```python
from build123d import *

# Parameters (mm, degrees)
BOSS_EXTRUDE1_DEPTH = 5
SKETCH2_R           = 2.5
CUT_EXTRUDE1_DEPTH  = 5
SKETCH3_R           = 3
CUT_EXTRUDE2_DEPTH  = 3
SKETCH4_R           = 2.5
BOSS_EXTRUDE2_DEPTH = 3


with BuildPart() as part:
    # Sketch1 → Boss-Extrude1 (new body)
    with BuildSketch(Plane.XY):
        Polygon((-87.5, 70), (-87.5, 65), (-92.5, 65), (-92.5, -65), (-87.5, -65), (-87.5, -70), (87.5, -70), (87.5, -65), (92.5, -65), (92.5, 65), (87.5, 65), (87.5, 70), align=None)
    extrude(amount=BOSS_EXTRUDE1_DEPTH)

    # Sketch2 → Cut-Extrude1 (cut)
    with BuildSketch(Plane.XY.offset(5)):
        with Locations((-52.5, -25)):
            Circle(SKETCH2_R)
        with Locations((-52.5, 25)):
            Circle(SKETCH2_R)
    extrude(amount=-CUT_EXTRUDE1_DEPTH, mode=Mode.SUBTRACT)

    # Sketch3 → Cut-Extrude2 (cut)
    with BuildSketch(Plane(origin=(0, 0, 0), x_dir=(-1, 0, 0), z_dir=(0, 0, -1))):
        with Locations((52.5, 25)):
            Circle(SKETCH3_R)
        with Locations((52.5, -25)):
            Circle(SKETCH3_R)
    extrude(amount=-CUT_EXTRUDE2_DEPTH, mode=Mode.SUBTRACT)

    # Sketch4 → Boss-Extrude2 (add)
    with BuildSketch(Plane.XY.offset(5)):
        with Locations(Location((58, 0, 0), (0, 0, 180))):
            Circle(SKETCH4_R)
        with BuildLine():
            Line((51.105600012, -5.785088487), (50.339555569, -6.427876097))
            ThreePointArc((50.339555569, -6.427876097), (58, -10), (65.660444431, -6.427876097))
            Line((65.660444431, -6.427876097), (64.894399988, -5.785088487))
            ThreePointArc((64.894399988, -5.785088487), (58, -9), (51.105600012, -5.785088487))
        make_face()
        with BuildLine():
            Line((68.724622204, -8.999026536), (69.490666647, -9.641814145))
            ThreePointArc((69.490666647, -9.641814145), (58, -15), (46.509333353, -9.641814145))
            Line((46.509333353, -9.641814145), (47.275377796, -8.999026536))
            ThreePointArc((47.275377796, -8.999026536), (58, -14), (68.724622204, -8.999026536))
        make_face()
        with BuildLine():
            Line((43.445155581, 12.212964584), (42.679111138, 12.855752194))
            ThreePointArc((42.679111138, 12.855752194), (58, 20), (73.320888862, 12.855752194))
            Line((73.320888862, 12.855752194), (72.554844419, 12.212964584))
            ThreePointArc((72.554844419, 12.212964584), (58, 19), (43.445155581, 12.212964584))
        make_face()
        with BuildLine():
            Line((47.275377796, 8.999026536), (46.509333353, 9.641814145))
            ThreePointArc((46.509333353, 9.641814145), (58, 15), (69.490666647, 9.641814145))
            Line((69.490666647, 9.641814145), (68.724622204, 8.999026536))
            ThreePointArc((68.724622204, 8.999026536), (58, 14), (47.275377796, 8.999026536))
        make_face()
        with BuildLine():
            Line((51.105600012, 5.785088487), (50.339555569, 6.427876097))
            ThreePointArc((50.339555569, 6.427876097), (58, 10), (65.660444431, 6.427876097))
            Line((65.660444431, 6.427876097), (64.894399988, 5.785088487))
            ThreePointArc((64.894399988, 5.785088487), (58, 9), (51.105600012, 5.785088487))
        make_face()
        with BuildLine():
            Line((43.445155581, -12.212964584), (42.679111138, -12.855752194))
            ThreePointArc((42.679111138, -12.855752194), (58, -20), (73.320888862, -12.855752194))
            Line((73.320888862, -12.855752194), (72.554844419, -12.212964584))
            ThreePointArc((72.554844419, -12.212964584), (58, -19), (43.445155581, -12.212964584))
        make_face()
    extrude(amount=BOSS_EXTRUDE2_DEPTH)


solid = part.part
```
Input: part model. Units: mm. Frame: model coordinates. A direction names the side the tool comes from. Give positions to 0.01 mm unless a question says otherwise; leave off trailing zeros. Order: outer loops, then holes, each group sorted by start corner. A loop starts at its lowest first (then second) coordinate and runs counter-clockwise, first axis right, second up. Notation, with made-up numbers: M 71,15 L 112,15 A31 ccw 112,41 Z; hole C 83.5,43.5 d7. An arc over 180 degrees is marked long. Return JSON: item names as keys, results as strings.
Item 1: Pull-direction query (Y, two-part tool) for faces 1 (the flat face through (-90, -65, 2)), 2 (the flat face through (87.5, -68, 2)), 3 (the cylindrical face through (-49.5, 25.1, 1.5)); classes: +Y half, -Y half, draft (parallel to the pull), parting line (faces both ways), or undercut.
Solutions:
{"face 1": "-Y half", "face 2": "draft", "face 3": "undercut"}
Item 2: Cut plane C-C (z = 6.75). Return loops of the section in (x, y), then the cut area to 3 significant figures.
Solutions:
{"outline": "M 42.68,-12.86 A20 ccw 73.32,-12.86 L 72.55,-12.21 A19 cw 43.45,-12.21 Z; M 42.68,12.86 L 43.45,12.21 A19 cw 72.55,12.21 L 73.32,12.86 A20 ccw Z; M 46.51,-9.64 A15 ccw 69.49,-9.64 L 68.72,-9 A14 cw 47.28,-9 Z; M 46.51,9.64 L 47.28,9 A14 cw 68.72,9 L 69.49,9.64 A15 ccw Z; M 50.34,-6.43 A10 ccw 65.66,-6.43 L 64.89,-5.79 A9 cw 51.11,-5.79 Z; M 50.34,6.43 L 51.11,5.79 A9 cw 64.89,5.79 L 65.66,6.43 A10 ccw Z; C 58,0 d5", "area": "171 mm^2"}
Item 3: Access query for faces 4 (the flat face through (90, -65, 2)), 5 (the cylindrical face through (58, 20, 6)), 6 (the flat face through (87.5, 67, 2)), 7 (the cylindrical face through (58, -10, 6)), 8 (the flat face through (-87.5, -67, 2)). Directions: +Z, -Z, +X, -X, +Y, -Y. A direction counts if a zero-diameter tool reaches every point of the face in a straight line with its end or side. Return the directions, or none.
Solutions:
{"face 4": "+Z, -Z, +X, -Y", "face 5": "+Z, +Y", "face 6": "+Z, -Z, +X, +Y", "face 7": "+Z", "face 8": "+Z, -Z, -X, -Y"}
Item 4: Cut plane A-A (y = 25). Return loops of the section in (x, z), then the cut area to 3 significant figures.
Solutions:
{"outline": "M -92.5,0 L -55.5,0 L -55.5,3 L -55,3 L -55,5 L -92.5,5 Z; M -50,3 L -49.5,3 L -49.5,0 L 92.5,0 L 92.5,5 L -50,5 Z", "area": "897 mm^2"}
Item 5: Ray query, probe 1 along Y at (x, z) = (-52.5, 4.15); probe 2 along Y at (x, z) = (-52.5, 1.25); probe 3 along Z at (x, y) = (26.5, -0.5). Return the intervals inside material, ascending.
Solutions:
{"probe 1": "-70 to -27.5, -22.5 to 22.5, 27.5 to 70", "probe 2": "-70 to -28, -22 to 22, 28 to 70", "probe 3": "0 to 5"}
Item 6: Cut plane B-B (x = -52.5). Return loops of the section in (y, z), then the cut area to 3 significant figures.
Solutions:
{"outline": "M -70,0 L -28,0 L -28,3 L -27.5,3 L -27.5,5 L -70,5 Z; M -22.5,3 L -22,3 L -22,0 L 22,0 L 22,3 L 22.5,3 L 22.5,5 L -22.5,5 Z; M 27.5,3 L 28,3 L 28,0 L 70,0 L 70,5 L 27.5,5 Z", "area": "644 mm^2"}
Item 7: First-contact query: P1, Ø1.5, axis at x = 91, z = 3.5, coming from the -Y side; P2, Ø2.5, axis at x = 90, z = 3.5, coming from the +Y side; P3, Ø1, axis at x = -58.5, y = 5, coming from the +Z side. Flat tips, straight axial feed; report the tip coordinate or a pass-through.
Solutions:
{"P1": "y = -65", "P2": "y = 65", "P3": "z = 5"}
